Work out the finished part from the listing and answer in its coordinate system (mm). Face numbers are marked on the shaded views. Round coordinates to 2 decimals unless told otherwise and drop trailing zeros. Order: outer loops, then holes, each group sorted by start corner. A loop starts at its lowest first (then second) coordinate and runs counter-clockwise, first axis right, second up. Notation, with made-up numbers: (59, 55) - (65, 55) arc R15 ccw to (65, 67) - close; hole circle Ø7 at (13.25, -12.75). An arc over 180 degrees is marked (long way). One line per question, with ' | ' between items. Start each with the question number.
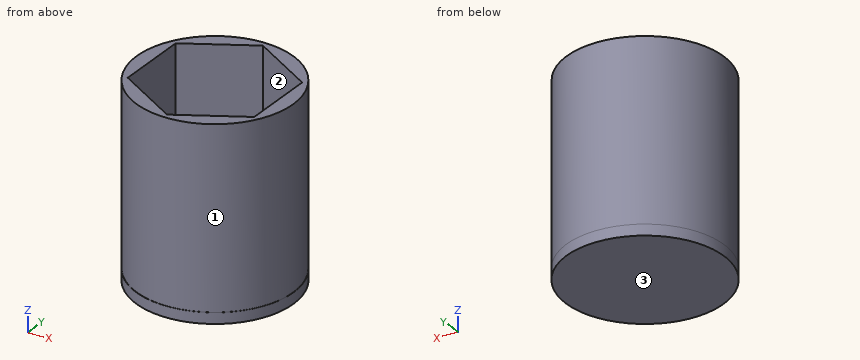
from build123d import *

# Parameters (mm, degrees)
F0_R     = 7.87972
F1_DEPTH = 18
F2_R     = 7.901402
F3_DEPTH = 1.1


with BuildPart() as f1:
    # F0 (on Top) → F1 (new body)
    with BuildSketch(Plane.XY):
        Circle(F0_R)
        Polygon((0, 7.366667), (6.37972, 3.683333), (6.37972, -3.683333), (0, -7.366667), (-6.37972, -3.683333), (-6.37972, 3.683333), align=None, mode=Mode.SUBTRACT)
    extrude(amount=F1_DEPTH)

    # F2 (on Top) → F3 (join)
    with BuildSketch(Plane.XY):
        Circle(F2_R)
    extrude(amount=-F3_DEPTH)


solid = f1.part
1) Straight lines are drawn through the part: line 1 (X direction, y = 0.25, z = 0.75); line 2 (X direction, y = 0.75, z = 1.75); line 3 (Y direction, x = -4.5, z = 5). For each, find the intervals that lie inside material, in ascending order.
2) Flat-ended cylindrical pins translate along their axes: pin 1 (5 mm diameter, centred on x = 0.5, y = 0, fed in from +Z); pin 2 (5 mm diameter, centred on x = 4.5, z = 12, fed in from -Y); pin 3 (6 mm diameter, centred on x = 3.5, z = 11.5, fed in from +Y). Find the tip coordinate at first contact, or state that the pin passes through.
3) Section A-A on z = 5.25 is taken. Give the vertices of the cut face in (x, y).
4) Determine the mould class of the marked faces 1, 2 and 3 for opening direction X: released by +X, released by -X, zero draft, split by the parting line, or undercut.
Recorded:
1) line 1: x = -7.88 to -6.38, 6.38 to 7.88 | line 2: x = -7.84 to -6.38, 6.38 to 7.84 | line 3: y = -6.47 to -4.77, 4.77 to 6.47
2) pin 1: stops at z = 0 | pin 2: stops at y = -7.62 | pin 3: stops at y = 7.86
3) outline: circle Ø15.76 at (0, 0); hole (-6.38, -3.68) - (0, -7.37) - (6.38, -3.68) - (6.38, 3.68) - (0, 7.37) - (-6.38, 3.68) - close
4) face 1: split by the parting line | face 2: undercut | face 3: zero draft
